from build123d import *

# Parameters (mm, degrees)
SKETCH1_R           = 2.6035
BOSS_EXTRUDE1_DEPTH = 107.95


with BuildPart() as part:
    # Sketch1 → Boss-Extrude1 (new body)
    with BuildSketch(Plane(origin=(0, 0, -152.4), x_dir=(-1, 0, 0), z_dir=(0, 0, -1))):
        with BuildLine():
            Line((6.416409763, -10.4902), (4.28752, -10.4902))
            ThreePointArc((4.28752, -10.4902), (3.545750844, -10.797450844), (3.2385, -11.53922))
            Line((3.2385, -11.53922), (3.2385, -11.65098))
            ThreePointArc((3.2385, -11.65098), (3.545750844, -12.392749156), (4.28752, -12.7))
            Line((4.28752, -12.7), (5.3170836, -12.7))
            ThreePointArc((5.3170836, -12.7), (5.8250836, -12.192), (6.3330836, -12.7))
            Line((6.3330836, -12.7), (9.5504, -12.7))
            ThreePointArc((9.5504, -12.7), (10.058323491, -12.192000006), (10.566399977, -12.699846982))
            ThreePointArc((10.566399977, -12.699846982), (12.082522516, -12.082522516), (12.699846982, -10.566399977))
            ThreePointArc((12.699846982, -10.566399977), (12.192000006, -10.058323491), (12.7, -9.5504))
            Line((12.7, -9.5504), (12.7, -6.3330836))
            ThreePointArc((12.7, -6.3330836), (12.192, -5.8250836), (12.7, -5.3170836))
            Line((12.7, -5.3170836), (12.7, 5.3171344))
            ThreePointArc((12.7, 5.3171344), (12.192, 5.8251344), (12.7, 6.3331344))
            Line((12.7, 6.3331344), (12.7, 9.5504))
            ThreePointArc((12.7, 9.5504), (12.192000006, 10.058323491), (12.699846982, 10.566399977))
            ThreePointArc((12.699846982, 10.566399977), (12.082522516, 12.082522516), (10.566399977, 12.699846982))
            ThreePointArc((10.566399977, 12.699846982), (10.058323491, 12.192000006), (9.5504, 12.7))
            Line((9.5504, 12.7), (6.3331344, 12.7))
            ThreePointArc((6.3331344, 12.7), (5.8251344, 12.192), (5.3171344, 12.7))
            Line((5.3171344, 12.7), (4.2874692, 12.7))
            ThreePointArc((4.2874692, 12.7), (3.545700044, 12.392749156), (3.2384492, 11.65098))
            Line((3.2384492, 11.65098), (3.2384492, 11.53922))
            ThreePointArc((3.2384492, 11.53922), (3.545700044, 10.797450844), (4.2874692, 10.4902))
            Line((4.2874692, 10.4902), (6.416384363, 10.4902))
            ThreePointArc((6.416384363, 10.4902), (7.355223148, 9.862578342), (7.134149423, 8.755124678))
            Line((7.134149423, 8.755124678), (3.796632915, 5.423689619))
            ThreePointArc((3.796632915, 5.423689619), (2.767299421, 4.736928798), (1.553617102, 4.4958))
            Line((1.553617102, 4.4958), (-1.657299581, 4.4958))
            ThreePointArc((-1.657299581, 4.4958), (-2.8709819, 4.736928798), (-3.900315394, 5.423689619))
            Line((-3.900315394, 5.423689619), (-7.207191475, 8.724540082))
            ThreePointArc((-7.207191475, 8.724540082), (-7.43216212, 9.851515102), (-6.476774195, 10.4902))
            Line((-6.476774195, 10.4902), (-4.2874692, 10.4902))
            ThreePointArc((-4.2874692, 10.4902), (-3.545700044, 10.797450844), (-3.2384492, 11.53922))
            Line((-3.2384492, 11.53922), (-3.2384492, 11.65098))
            ThreePointArc((-3.2384492, 11.65098), (-3.545700044, 12.392749156), (-4.2874692, 12.7))
            Line((-4.2874692, 12.7), (-5.3170836, 12.7))
            ThreePointArc((-5.3170836, 12.7), (-5.8250836, 12.192), (-6.3330836, 12.7))
            Line((-6.3330836, 12.7), (-9.5504, 12.7))
            ThreePointArc((-9.5504, 12.7), (-10.058323491, 12.192000006), (-10.566399977, 12.699846982))
            ThreePointArc((-10.566399977, 12.699846982), (-12.082522516, 12.082522516), (-12.699846982, 10.566399977))
            ThreePointArc((-12.699846982, 10.566399977), (-12.192000006, 10.058323491), (-12.7, 9.5504))
            Line((-12.7, 9.5504), (-12.7, 6.3331344))
            ThreePointArc((-12.7, 6.3331344), (-12.192, 5.8251344), (-12.7, 5.3171344))
            Line((-12.7, 5.3171344), (-12.7, 4.287470133))
            ThreePointArc((-12.7, 4.287470133), (-12.392749156, 3.545700977), (-11.65098, 3.238450133))
            Line((-11.65098, 3.238450133), (-11.53922, 3.238450133))
            ThreePointArc((-11.53922, 3.238450133), (-10.797450844, 3.545700977), (-10.4902, 4.287470133))
            Line((-10.4902, 4.287470133), (-10.4902, 6.402089023))
            ThreePointArc((-10.4902, 6.402089023), (-9.856394933, 7.351113629), (-8.736962546, 7.129240479))
            Line((-8.736962546, 7.129240479), (-5.440484187, 3.838768792))
            ThreePointArc((-5.440484187, 3.838768792), (-4.75073678, 2.808015636), (-4.5085, 1.591658411))
            Line((-4.5085, 1.591658411), (-4.5085, -1.591658411))
            ThreePointArc((-4.5085, -1.591658411), (-4.75073678, -2.808015636), (-5.440484187, -3.838768792))
            Line((-5.440484187, -3.838768792), (-8.736962546, -7.129240479))
            ThreePointArc((-8.736962546, -7.129240479), (-9.856394933, -7.351113629), (-10.4902, -6.402089023))
            Line((-10.4902, -6.402089023), (-10.4902, -4.287470133))
            ThreePointArc((-10.4902, -4.287470133), (-10.797450844, -3.545700977), (-11.53922, -3.238450133))
            Line((-11.53922, -3.238450133), (-11.65098, -3.238450133))
            ThreePointArc((-11.65098, -3.238450133), (-12.392749156, -3.545700977), (-12.7, -4.287470133))
            Line((-12.7, -4.287470133), (-12.7, -5.3170836))
            ThreePointArc((-12.7, -5.3170836), (-12.192, -5.8250836), (-12.7, -6.3330836))
            Line((-12.7, -6.3330836), (-12.7, -9.5504))
            ThreePointArc((-12.7, -9.5504), (-12.192000006, -10.058323491), (-12.699846982, -10.566399977))
            ThreePointArc((-12.699846982, -10.566399977), (-12.082522516, -12.082522516), (-10.566399977, -12.699846982))
            ThreePointArc((-10.566399977, -12.699846982), (-10.058323491, -12.192000006), (-9.5504, -12.7))
            Line((-9.5504, -12.7), (-6.3331344, -12.7))
            ThreePointArc((-6.3331344, -12.7), (-5.8251344, -12.192), (-5.3171344, -12.7))
            Line((-5.3171344, -12.7), (-4.28752, -12.7))
            ThreePointArc((-4.28752, -12.7), (-3.545750844, -12.392749156), (-3.2385, -11.65098))
            Line((-3.2385, -11.65098), (-3.2385, -11.53922))
            ThreePointArc((-3.2385, -11.53922), (-3.545750844, -10.797450844), (-4.28752, -10.4902))
            Line((-4.28752, -10.4902), (-6.40834956, -10.4902))
            ThreePointArc((-6.40834956, -10.4902), (-7.350269456, -9.860518594), (-7.128470204, -8.749430454))
            Line((-7.128470204, -8.749430454), (-3.796658315, -5.423689619))
            ThreePointArc((-3.796658315, -5.423689619), (-2.767324821, -4.736928798), (-1.553642502, -4.4958))
            Line((-1.553642502, -4.4958), (1.553642502, -4.4958))
            ThreePointArc((1.553642502, -4.4958), (2.767324821, -4.736928798), (3.796658315, -5.423689619))
            Line((3.796658315, -5.423689619), (7.134174823, -8.755124678))
            ThreePointArc((7.134174823, -8.755124678), (7.355248548, -9.862578342), (6.416409763, -10.4902))
        make_face()
        Circle(SKETCH1_R, mode=Mode.SUBTRACT)
        with BuildLine():
            Line((10.4902, 6.446436794), (10.4902, -6.425372487))
            ThreePointArc((10.4902, -6.425372487), (9.862352148, -7.36547709), (8.753441447, -7.145689354))
            Line((8.753441447, -7.145689354), (5.440484187, -3.838768792))
            ThreePointArc((5.440484187, -3.838768792), (4.75073678, -2.808015636), (4.5085, -1.591658411))
            Line((4.5085, -1.591658411), (4.5085, 1.591658411))
            ThreePointArc((4.5085, 1.591658411), (4.75073678, 2.808015636), (5.440484187, 3.838768792))
            Line((5.440484187, 3.838768792), (8.768349738, 7.160570479))
            ThreePointArc((8.768349738, 7.160570479), (9.867741577, 7.378471563), (10.4902, 6.446436794))
        make_face(mode=Mode.SUBTRACT)
    extrude(amount=-BOSS_EXTRUDE1_DEPTH)


solid = part.part
Geometry: final body of the model. Coordinates: model frame, mm. A direction names the side the tool comes from. Coordinates: 2 decimals unless noted, no trailing zeros. Loops run counter-clockwise (first coordinate to the right, second up) from the corner with the lowest first, then second, coordinate; pieces in that order, holes last. Notation, with made-up numbers: M 80,89 L 132,89 A17 ccw 132,106 Z; hole C -20,85.5 d8. An arc over 180 degrees is marked long. One line per item, written item: value. Start each with the question number.
1) Cut plane C-C (z = -118). Count the separate pieces of the cut face and the enclosed holes in it, then the cut area to 3 significant figures.
2) Draft query along Y for faces 4 (the flat face through (8, 12.7, -99)), 5 (the flat face through (-10.49, 0, -99)), 6 (the flat face through (-3, 0, -152.4)). Return one class per face: released by +Y, released by -Y, zero draft, split by the parting line, or undercut.
3) Cut plane B-B (x = 0). Return loops of the section in (y, z), then the cut area to 3 significant figures.
4) Cut plane A-A (y = 0). Return loops of the section in (x, z), then the cut area to 3 significant figures.
5) Material intervals for L1, parallel to X at y = 0.25, z = -90.5; L2, parallel to X at y = -9.5, z = -127; L3, parallel to Y at x = 0, z = -97.5, sorted ascending. Write a range as from..to.
6) Reachability of faces 1 (the flat face through (-3, 0, -44.45)), 2 (the flat face through (4.508, 0, -99)), 3 (the cylindrical face through (4.744, -2.792, -99.181)) from +Z, -Z, +X, -X, +Y, -Y: full face, straight path, thin tool, end or side. Return the list, or none.
7) Pin query (flat end, axial travel): P1, Ø1, axis at x = 0.5, z = -78.5, coming from the +Y side; P2, Ø1.6, axis at y = -0.5, z = -79.5, coming from the +X side; P3, Ø4, axis at y = 1.5, z = -94.5, coming from the +X side. Return the tip coordinate at first contact, or that it passes through.
Evaluation:
1. separate pieces: 1
1. enclosed holes: 2
1. area: 297 mm^2
2. face 4: released by +Y
2. face 5: undercut
2. face 6: zero draft
3. outline: M -4.5,-152.4 L -2.6,-152.4 L -2.6,-44.45 L -4.5,-44.45 Z; M 2.6,-152.4 L 4.5,-152.4 L 4.5,-44.45 L 2.6,-44.45 Z
3. area: 409 mm^2
4. outline: M -12.7,-152.4 L -10.49,-152.4 L -10.49,-44.45 L -12.7,-44.45 Z; M -4.51,-152.4 L -2.6,-152.4 L -2.6,-44.45 L -4.51,-44.45 Z; M 2.6,-152.4 L 4.51,-152.4 L 4.51,-44.45 L 2.6,-44.45 Z
4. area: 650 mm^2
5. L1: -12.7..-10.49, -4.51..-2.59, 2.59..4.51
5. L2: -12.7..-7.43, 7.43..12.7
5. L3: -4.5..-2.6, 2.6..4.5
6. face 1: +Z, +X, -X, +Y, -Y
6. face 2: +Z, -Z, +X
6. face 3: +Z, -Z
7. P1: y = 4.5
7. P2: x = 4.51
7. P3: x = 12.34
